The model under review builds one solid part; all positions refer to its coordinate system, in mm. A direction names the side the tool comes from. Give positions to 0.01 mm unless a question says otherwise; leave off trailing zeros. Order: outer loops, then holes, each group sorted by start corner. A loop starts at its lowest first (then second) coordinate and runs counter-clockwise, first axis right, second up. Notation, with made-up numbers: (35, 70) -> (41, 70) arc R15 cw to (41, 74) -> close; hole circle Ø9 at (78.5, 38.5). An arc over 180 degrees is marked (long way). Use one line per item in the form item = value.
```python
from build123d import *

# Parameters (mm, degrees)
F1_DEPTH = 15
F3_DEPTH = 40


with BuildPart() as f1:
    # F0 (on Front) → F1 (new body)
    with BuildSketch(Plane.XZ):
        Polygon((0, 40), (0, 0), (50, 0), align=None)
    extrude(amount=F1_DEPTH)

    # F2 (on Top) → F3 (join)
    with BuildSketch(Plane.XY):
        Polygon((0, 50), (0, 0), (50, 0), (50, 24.924569), (80, 25), (80, 50), align=None)
    extrude(amount=F3_DEPTH)


solid = f1.part
```
1. Add section D-D on z = 31. Give the boundary of the cut face in (x, y), then the cut area to 3 significant figures.
Values:
outline = (0, -15) -> (11.25, -15) -> (11.25, 0) -> (50, 0) -> (50, 24.92) -> (80, 25) -> (80, 50) -> (0, 50) -> close
area = 3,420 mm^2
2. For L1, parallel to X at y = 18, z = 36; L2, parallel to Y at x = 53.5, z = 37, list the stretches that pass through material, from the lowest coordinate up.
Values:
L1 = 0 to 50
L2 = 24.93 to 50
3. Add section B-B on x = 36. Give the boundary of the cut face in (y, z), then the cut area to 3 significant figures.
Values:
outline = (-15, 0) -> (50, 0) -> (50, 40) -> (0, 40) -> (0, 11.2) -> (-15, 11.2) -> close
area = 2,170 mm^2
4. For pin 1 Ø2 at (y, z) = (0, 7) entering from +X; pin 2 Ø4 at (x, z) = (64, 22.5) entering from -Y; pin 3 Ø3 at (y, z) = (3, 4.5) entering from -X, all flat-tipped, find the tip position at first contact; note any pin that passes through.
Values:
pin_1 = 50
pin_2 = 24.95
pin_3 = 0
5. Add section A-A on z = 16. Give the boundary of the cut face in (x, y), then the cut area to 3 significant figures.
Values:
outline = (0, -15) -> (30, -15) -> (30, 0) -> (50, 0) -> (50, 24.92) -> (80, 25) -> (80, 50) -> (0, 50) -> close
area = 3,700 mm^2
6. Tool access review of faces 1 (the face through (31, 18, 0)), 2 (the face through (50, 12, 20)), 3 (the face through (25, -7, 20)): name each direction out of +Z, -Z, +X, -X, +Y, -Y from which nothing blocks a thin tool from reaching the whole face with its end or side.
Values:
face_1 = -Z, +X, -X, +Y, -Y
face_2 = +Z, -Z, +X, -Y
face_3 = +Z, +X, -Y
7. Add section C-C on y = 7.5. Give the boundary of the cut face in (x, z), then the cut area to 3 significant figures.
Values:
outline = (0, 0) -> (50, 0) -> (50, 40) -> (0, 40) -> close
area = 2,000 mm^2
